Geometry: final body of the model. Coordinates: model frame, mm. A direction names the side the tool comes from. Give positions to 0.01 mm unless a question says otherwise; leave off trailing zeros. Write each loop counter-clockwise with the first axis right and the second up, starting at its lowest first coordinate (ties: lowest second). Pieces come first, ordered by that corner, then holes.
Q1. Reachability of faces 4 (the face through (-187, 100, -52)), 5 (the face through (137, -50, -52)), 6 (the face through (-75, 51, 7)), 7 (the face through (125, -38, -52)) from +Z, -Z, +X, -X, +Y, -Y: full face, straight path, thin tool, end or side. Return the list, or none.
Q2. Cut plane D-D on y = 107. Return the cut outline in (x, z).
Q3. Cut plane A-A on z = -70.5. Return the cut outline in (x, y).
Q4. Cut plane B-B on x = -93. Return the cut outline in (y, z).
Q5. Cut plane C-C on x = 145. Return the cut outline in (y, z).
Q6. Draft query along X for faces 1 (the face through (137, -37, -105)), 2 (the face through (-175, -7, 7)), 3 (the face through (-175, -38, -52)). Return one class per face: pulls with the +X half, pulls with the -X half, needs draft (parallel to the pull), parting line crosses it, or undercut.
Q7. Pin query (flat end, axial travel): pin 1 (7.5 mm diameter, centred on x = -190, z = -68.5, fed in from -Y); pin 2 (3 mm diameter, centred on x = 99, y = -12, fed in from -Z); pin 3 (12.5 mm diameter, centred on x = 131.5, z = -69, fed in from +Y). Return the tip coordinate at first contact, or that it passes through.
Q8. Line query: L1, parallel to X at y = 79, z = -88; L2, parallel to Y at x = -181.5, z = -14.5; L3, parallel to Z at x = 159.5, y = -85. Output: solid intervals per line, ascending.
```python
from build123d import *

# Parameters (mm, degrees)
F0_W     = 25
F0_H     = 25
F1_DEPTH = 15
F2_DEPTH = 105
F3_DEPTH = 15


with BuildPart() as f1:
    # F0 (on Top) → F1 (new body)
    with BuildSketch(Plane.XY):
        Polygon((200, 150), (-200, 150), (-200, 100), (-175, 100), (-175, 90), (-160, 90), (-75, 90), (-75, 10), (-160, 10), (-175, 10), (-175, -25), (-175, -50), (-200, -50), (-200, -150), (200, -150), align=None)
        with Locations((137.5, -37.5)):
            Rectangle(F0_W, F0_H, mode=Mode.SUBTRACT)
        with Locations((137.5, 87.5)):
            Rectangle(F0_W, F0_H, mode=Mode.SUBTRACT)
    extrude(amount=F1_DEPTH)

    # F0 (on Top) → F2 (join)
    with BuildSketch(Plane.XY):
        Polygon((-175, 100), (-200, 100), (-200, 75), (-175, 75), (-175, 90), align=None)
        with Locations((-187.5, -37.5)):
            Rectangle(F0_W, F0_H)
        with Locations((137.5, -37.5)):
            Rectangle(F0_W, F0_H)
        with Locations((137.5, 87.5)):
            Rectangle(F0_W, F0_H)
    extrude(amount=-F2_DEPTH)

    # F0 (on Top) → F3 (join)
    with BuildSketch(Plane.XY):
        with Locations((137.5, 87.5)):
            Rectangle(F0_W, F0_H)
        with Locations((137.5, -37.5)):
            Rectangle(F0_W, F0_H)
        with Locations((-187.5, -37.5)):
            Rectangle(F0_W, F0_H)
        Polygon((-175, 100), (-200, 100), (-200, 75), (-175, 75), (-175, 90), align=None)
    extrude(amount=F3_DEPTH)


solid = f1.part
```
Data:
1. face 4: -Z, +X, -X, +Y
1. face 5: -Z, +X, -X, -Y
1. face 6: +Z, -Z
1. face 7: -Z, +Y, -Y
2. outline: (-200, 0) - (200, 0) - (200, 15) - (-200, 15) - close
3. outline: (-200, -50) - (-175, -50) - (-175, -25) - (-200, -25) - close; (-200, 75) - (-175, 75) - (-175, 100) - (-200, 100) - close; (125, -50) - (150, -50) - (150, -25) - (125, -25) - close; (125, 75) - (150, 75) - (150, 100) - (125, 100) - close
4. outline: (-150, 0) - (10, 0) - (10, 15) - (-150, 15) - close; (90, 0) - (150, 0) - (150, 15) - (90, 15) - close
5. outline: (-150, 0) - (-50, 0) - (-50, -105) - (-25, -105) - (-25, 0) - (75, 0) - (75, -105) - (100, -105) - (100, 0) - (150, 0) - (150, 15) - (-150, 15) - close
6. face 1: needs draft
6. face 2: pulls with the -X half
6. face 3: undercut
7. pin 1: stops at y = -50
7. pin 2: stops at z = 0
7. pin 3: stops at y = 100
8. L1: x = -200 to -175, 125 to 150
8. L2: y = -50 to -25, 75 to 100
8. L3: z = 0 to 15
